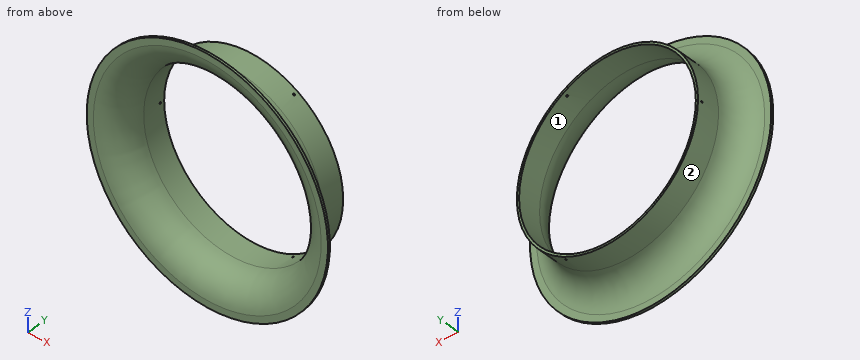
```python
from build123d import *

# Parameters (mm, degrees)
LOFT_THIN1_START       = 39
LOFT_THIN1_OUTLINE_R   = 205
LOFT_THIN1_OUTLINE_R_2 = 200
LOFT_THIN1_DEPTH       = 52
SKETCH6_R              = 2
CUT_EXTRUDE1_DEPTH     = 10
CIRPATTERN1_COUNT      = 3


# Read off the part's stored shape, not the designer's step: Loft-Thin1
with BuildPart() as part:
    # Loft-Thin1 outline → Loft-Thin1 (new body)
    with BuildSketch(Plane(origin=(0, 0, 0), x_dir=(1, 0, 0), z_dir=(0, 1, 0)).offset(LOFT_THIN1_START)):
        Circle(LOFT_THIN1_OUTLINE_R)
        Circle(LOFT_THIN1_OUTLINE_R_2, mode=Mode.SUBTRACT)
    extrude(amount=LOFT_THIN1_DEPTH)

    # Sketch5 → Revolve-Thin2 (revolve)
    with BuildSketch(Plane.XY, mode=Mode.PRIVATE) as revolve_thin2_sk:
        with BuildLine():
            ThreePointArc((205, 39), (220.240453532, -0.187002767), (257.952454685, -18.779947095))
            Line((257.952454685, -18.779947095), (272.952454685, -18.779947095))
            Line((272.952454685, -18.779947095), (272.952454685, -23.779947095))
            Line((272.952454685, -23.779947095), (257.738988428, -23.779947095))
            ThreePointArc((257.738988428, -23.779947095), (216.629515158, -3.647135138), (200, 39))
            Line((200, 39), (205, 39))
        make_face()
    revolve(revolve_thin2_sk.sketch.rotate(Axis((0, 91, 0), (0, -1, 0)), 90), axis=Axis((0, 91, 0), (0, -1, 0)))

    # Sketch6 → Cut-Extrude1 (cut)
    with BuildSketch(Plane.ZY.offset(205)):
        with Locations((0, 81)):
            Circle(SKETCH6_R)
    cut_extrude1 = extrude(amount=-CUT_EXTRUDE1_DEPTH, mode=Mode.SUBTRACT)

    # CirPattern1: Cut-Extrude1 ×3 about axis
    cirpattern1_axis = Axis((0, 91, 0), (0, 1, 0))
    for i in range(1, CIRPATTERN1_COUNT):
        add(cut_extrude1.rotate(cirpattern1_axis, i * 360 / CIRPATTERN1_COUNT), mode=Mode.SUBTRACT)


solid = part.part
```
The model under review builds one solid part; all positions refer to its coordinate system, in mm. Face numbers are marked on the shaded views. Coordinates: 2 decimals unless noted, no trailing zeros. Write each loop counter-clockwise with the first axis right and the second up, starting at its lowest first coordinate (ties: lowest second). Pieces come first, ordered by that corner, then holes. Notation, with made-up numbers: (69.5, 89.25) - (88.5, 89.25) arc R26 cw to (88.5, 127.25) - close; hole circle Ø11 at (-15.5, 70). An arc over 180 degrees is marked (long way). Answer in a Markdown table with one row per item. Add a question column.
Q1. Consider section A-A on x = 0. Give the boundary of the cut face in (y, z), then the cut area to 3 significant figures.
Q2. Consider section C-C on y = -11. Give the boundary of the cut face in (x, z), then the cut area to 3 significant figures.
Q3. Draft analysis for pull direction Z (two halves, no side actions). For the marked faces 1 and 2, state which applies: +Z half, -Z half, draft (parallel to the pull), parting line (faces both ways), or undercut.
Q4. To check wall thickness, follow line 1 along X through (y, z) = (63, 0); line 2 along Y through (x, z) = (-149.5, -226.5). State the ranges of each line that lie inside material, in increasing order. Write a range as from..to.
Q5. Consider section B-B on y = 68. Give the boundary of the cut face in (x, z), then the cut area to 3 significant figures.
Q6. Clearance check with flat-ended pins moving along their axes: pin 1 (12 mm diameter, centred on y = 72.5, z = -163.5, fed in from -X); pin 2 (2 mm diameter, centred on x = 110, z = -178, fed in from -Y); pin 3 (10 mm diameter, centred on y = 64, z = -50.5, fed in from +X). State where each tip first meets the part, or that it passes through.
Answers below:
| question | item | result |
|---|---|---|
| 1 | outline | (-23.78, -272.95) - (-18.78, -272.95) - (-18.78, -257.95) arc R58 cw to (39, -205) - (91, -205) - (91, -200) - (39, -200) arc R63 ccw to (-23.78, -257.74) - close; (-23.78, 257.74) arc R63 ccw to (39, 200) - (91, 200) - (91, 205) - (39, 205) arc R58 cw to (-18.78, 257.95) - (-18.78, 272.95) - (-23.78, 272.95) - close |
| 1 | area | 1,570 mm² |
| 2 | outline | circle Ø467.21 at (0, 0); hole circle Ø449.34 at (0, 0) |
| 2 | area | 12,900 mm² |
| 3 | face 1 | undercut |
| 3 | face 2 | parting line |
| 4 | line 1 | -205..-200, 200..205 |
| 4 | line 2 | -23.78..-18.78 |
| 5 | outline | circle Ø410 at (0, 0); hole circle Ø400 at (0, 0) |
| 5 | area | 6,360 mm² |
| 6 | pin 1 | x = -131.22 |
| 6 | pin 2 | y = 4.56 |
| 6 | pin 3 | x = 199.89 |
